Part model, mm, in its own coordinate system. A direction names the side the tool comes from. Coordinates: 2 decimals unless noted, no trailing zeros. Loops run counter-clockwise (first coordinate to the right, second up) from the corner with the lowest first, then second, coordinate; pieces in that order, holes last. Notation, with made-up numbers: M -38,21.5 L -3,21.5 A29 cw -3,58.5 Z; hole C 2,34.5 d2. An arc over 180 degrees is marked long. Answer as a JSON object with one key per item and string values. Group by question number.
1. Saw through at C-C on y = 11. Write the cut outline in (x, z).
2. Drill centre lines: L1, parallel to Z at x = -24, y = 11.25; L2, parallel to Z at x = 24, y = 11.4; L3, parallel to Z at x = -14.5, y = 1.5. Where is each one in solid material? Low to high.
3. Drop flat-ended pins along their axis: pin 1 Ø3 at (x, z) = (24, 10.77) entering from -Y; pin 2 Ø8 at (x, y) = (-11.5, -5.5) entering from +Z; pin 3 Ø8 at (y, z) = (-5, 7) entering from +X; pin 4 Ø8 at (y, z) = (1.5, 6) entering from +X. Give the stop position or say it passes through.
4. Saw through at D-D on x = -23.5. Write the cut outline in (y, z).
5. 3-axis set-ups, long thin cutter, end or side, ignore diameter. For faces 1 (the face through (20.5, 12, 11)), 2 (the face through (24, 10.35, 13)), 3 (the face through (0, 0, 0)): which of +Z, -Z, +X, -X, +Y, -Y reach the whole face in a straight line?
6. Saw through at A-A on z = 8.5. Write the cut outline in (x, y), then the cut area to 3 significant figures.
7. Saw through at B-B on y = 0. Write the cut outline in (x, z).
8. Mould opens along Z. For faces 4 (the face through (-23.92, 11.66, 22.88)), 5 (the face through (27.5, 7, 2)), 6 (the face through (25.19, 11.66, 11.15)), 7 (the face through (24.672, 11.656, 20.434)) say: released by +Z, released by -Z, zero draft, split by the parting line, or undercut.
Autodesk Inventor part; units mm, degrees
ref_plane "YZ Plane" through (0, 0, 0) normal (1, 0, 0) x (0, 1, 0)
ref_plane "XZ Plane" through (0, 0, 0) normal (0, 1, 0) x (-1, 0, 0)
ref_plane "XY Plane" through (0, 0, 0) normal (0, 0, 1) x (1, 0, 0)
sketch "Base" plane through (0, 0, 0) normal (0, 0, 1) x (1, 0, 0)
  line L0 (27.5, -13) -> (-27.5, -13)
  line L1 (-27.5, -13) -> (-27.5, 13)
  line L2 (-27.5, 13) -> (27.5, 13)
  line L3 (27.5, 13) -> (27.5, -13)
  line L4 (27.5, -13) -> (-27.5, 13) construction
  line L5 (-27.5, -13) -> (27.5, 13) construction
  line L6 (-27.5, 0) -> (27.5, 0) construction
  circle A0 centre (-24.15, 0) radius 1.5
  line L7 (0, -18.2) -> (0, 18.2) construction
  line L8 (-25.65, -1.5) -> (-22.65, -1.5) construction
  line L9 (-22.65, -1.5) -> (-22.65, 1.5)
  line L10 (-22.65, 1.5) -> (-25.65, 1.5) construction
  line L11 (-25.65, 1.5) -> (-25.65, -1.5) construction
  line L12 (-25.65, -1.5) -> (-22.65, 1.5) construction
  line L13 (-22.65, -1.5) -> (-25.65, 1.5) construction
  circle A1 centre (24.15, 0) radius 1.5
  point P0 (0, 0)
  dimension "d0" = 55
  dimension "d1" = 26
  dimension "d4" = 3
  dimension "d5" = 1.85
extrude "BaseFeature" add sketch "Base" along normal blind 2.88
fillet "BaseFilletsFeature" radius 6 2 edges at (-27.5, -13, 1.44) (27.5, -13, 1.44)
sketch "ServoMount" plane through (0, 0, 2.88) normal (0, 0, 1) x (1, 0, 0)
  line L0 (27.5, 13) -> (-27.5, 13)
  line L1 (-27.5, 13) -> (-27.5, -7)
  line L2 (27.5, -7) -> (27.5, 13)
  line L3 (-27.5, 13) -> (-20.5, 13)
  line L4 (-20.5, 13) -> (-20.5, 10.35)
  line L5 (-20.5, 10.35) -> (-27.5, 10.35)
  line L6 (-27.5, 10.35) -> (-27.5, 13)
  line L7 (0, -18.2) -> (0, 18.2) construction
  line L8 (20.5, 13) -> (20.5, 10.35)
  line L9 (20.5, 10.35) -> (27.5, 10.35)
  point P0 (0, 0)
  point P1 (-24, 13)
  dimension "d7" = 2.65
  dimension "d8" = 7
extrude "ServoMountFEature" add sketch "ServoMount" along normal blind 20
sketch "ServoMountProfile" plane through (-27.5, 10.35, 2.88) normal (0, -1, 0) x (1, 0, 0)
  line L0 (7, 0) -> (0, 0)
  line L1 (7, 0) -> (7, 20)
  line L2 (0, 20) -> (7, 20)
  line L3 (0, 0) -> (0, 20)
  line L4 (27.5, -7.456) -> (27.5, 24.576) construction
  circle A0 centre (3.5, 16.5) radius 3.5
  line L5 (3.5, 20) -> (3.5, 0) construction
  line L6 (0, 20) -> (7, 20)
  line L7 (0, 0) -> (0, 20)
  circle A1 centre (51.5, 16.5) radius 3.5
  line L8 (48, 0) -> (48, 20)
  line L9 (48, 20) -> (55, 20)
  line L10 (55, 0) -> (55, 20)
  point P0 (27.5, -2.88)
  point P1 (55, 16.5)
  point P2 (51.5, 20)
  point P3 (48, 16.5)
  point P4 (0, 16.5)
  point P5 (3.5, 20)
  point P6 (7, 16.5)
extrude "ServoMountProfileFeature" cut sketch "ServoMountProfile" against normal blind 20 contours A0 L2 L1 | L3 L2 A0 | A1 L9 L10 | A1 L8 L9
sketch "ServoMountHoles" plane through (-27.5, 10.35, 2.88) normal (0, -1, 0) x (1, 0, 0)
  arc A0 (7, 16.5) -> (0, 16.5) centre (3.5, 16.5) ccw construction
  line L0 (0, 0) -> (0, 16.5) construction
  line L1 (7, 0) -> (0, 0) construction
  line L2 (7, 0) -> (7, 16.5) construction
  line L3 (27.5, 24.576) -> (27.5, -7.456) construction
  circle A1 centre (51.5, 16.5) radius 1.25
  circle A2 centre (51.5, 7.89) radius 1.25
  arc A3 (-3.5754, 4) -> (-3.5754, 7) centre (-2.2525, 5.5) ccw construction
  arc A4 (-3.5754, 15) -> (-3.5754, 18) centre (-2.2525, 16.5) ccw construction
  circle A5 centre (-2.2525, 5.5) radius 2
  arc A6 (7, 16.5) -> (0, 16.5) centre (3.5, 16.5) ccw
  circle A7 centre (3.5, 16.5) radius 2
  point P0 (27.5, -2.88)
  dimension "d17" = 4
  dimension "d18" = 4
extrude "ServoMountHolesFeature" cut sketch "ServoMountHoles" against normal through all
properties part number "M3RCServoMountBracket"
Outcome:
{
 "1": {"outline": "M -27.5,0 L 27.5,0 L 27.5,19.38 A3.5 ccw 20.5,19.38 L 20.5,2.88 L -20.5,2.88 L -20.5,19.38 A3.5 ccw -27.5,19.38 Z; hole C -24,19.38 d4; hole C 24,10.77 d2.5; hole C 24,19.38 d2.5"},
 "2": {"L1": "z = 0 to 17.38, 21.38 to 22.88", "L2": "z = 0 to 9.52, 12.02 to 18.13, 20.63 to 22.88", "L3": "z = 0 to 2.88"},
 "3": {"pin 1": "stops at y = 10.35", "pin 2": "stops at z = 2.88", "pin 3": "passes through", "pin 4": "stops at x = 27.5"},
 "4": {"outline": "M -12.66,0 L -1.35,0 L -1.35,2.88 L -12.66,2.88 Z; M 1.35,0 L 13,0 L 13,17.44 L 10.35,17.44 L 10.35,2.88 L 1.35,2.88 Z; M 10.35,21.32 L 13,21.32 L 13,22.84 L 10.35,22.84 Z"},
 "5": {"face 1": "+Z, +Y, -Y", "face 2": "+Z, +X, -X, -Y", "face 3": "-Z, +X, -X, +Y, -Y"},
 "6": {"outline": "M -27.5,10.35 L -20.5,10.35 L -20.5,13 L -27.5,13 Z; M 20.5,10.35 L 27.5,10.35 L 27.5,13 L 20.5,13 Z", "area": "37.1 mm²"},
 "7": {"outline": "M -27.5,0 L -25.65,0 L -25.65,2.88 L -27.5,2.88 Z; M -22.65,0 L 22.65,0 L 22.65,2.88 L -22.65,2.88 Z; M 25.65,0 L 27.5,0 L 27.5,2.88 L 25.65,2.88 Z"},
 "8": {"face 4": "released by +Z", "face 5": "zero draft", "face 6": "undercut", "face 7": "undercut"}
}
